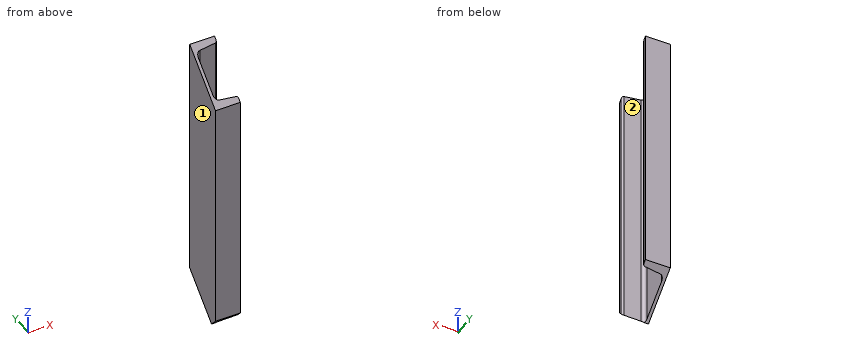
Autodesk Inventor part; units mm, degrees
ref_plane "Начальная плоскость" through (0, 0, 23.4485) normal (0, 0, 1) x (1, 0, 0)
ref_plane "Конечная плоскость" through (0, 0, 422.7409) normal (0, 0, 1) x (1, 0, 0)
ref_plane "РабПлоскость8" through (36, 285.6248, 665.6679) normal (0, -0.6924238, 0.721491) x (1, 0, 0)
ref_plane "Начальная плоскость" through (0, 0, 23.4485) normal (0, 0, 1) x (1, 0, 0)
ref_plane "Конечная плоскость" through (0, 0, 422.7409) normal (0, 0, 1) x (1, 0, 0)
sketch "Эскиз" plane through (0, 0, 0) normal (0, 0, 1) x (1, 0, 0)
  line L0 (36, -32.5) -> (0, -32.5)
  line L1 (36, -32.5) -> (36, -28.696)
  line L2 (33.6994, -26.2039) -> (9.9215, -24.3017)
  line L3 (4.4, -18.3208) -> (4.4, 18.3208)
  line L4 (33.6994, 26.2039) -> (9.9215, 24.3017)
  line L5 (36, 28.696) -> (36, 32.5)
  line L6 (0, 32.5) -> (36, 32.5)
  line L7 (0, -32.5) -> (0, 32.5)
  arc A0 (4.4, -18.3208) -> (9.9215, -24.3017) centre (10.4, -18.3208) ccw
  arc A1 (9.9215, 24.3017) -> (4.4, 18.3208) centre (10.4, 18.3208) ccw
  arc A2 (36, -28.696) -> (33.6994, -26.2039) centre (33.5, -28.696) ccw
  arc A3 (33.6994, 26.2039) -> (36, 28.696) centre (33.5, 28.696) ccw
  line L8 (0, 45.5) -> (0, -45.5) construction
  line L9 (-7.2974, 0) -> (43.7847, 0) construction
  point P0 (36, -26.388)
  point P1 (4.4, -23.86)
  point P2 (4.4, 23.86)
  point P3 (36, 26.388)
  dimension "d3" = 36
  dimension "d5" = 4.4
  dimension "d7" = 65
  dimension "d9" = 8.64
  dimension "d11" = 8.64
  dimension "d13" = 6.112
  dimension "d15" = 6.112
  dimension "d22" = 6
  dimension "d23" = 2.5
  dimension "d24" = 32.5
  dimension "d25" = 0
extrude "Тело" add sketch "Эскиз" along normal up to surface (399.2924 mm away) from surface at 23.4485
sketch "Sketch3" plane through (0, 0, 0) normal (0, 0, 1) x (1, 0, 0)
  line L0 (0, 0) -> (10, 0)
ref_plane "Work Plane7" through (0, 0, 0) normal (0, -1, 0) x (1, 0, 0)
sketch "Sketch4" plane through (0, 0, 0) normal (0, -1, 0) x (1, 0, 0)
  line L0 (-2, 23.4485) -> (12, 23.4485)
  line L1 (-2, 422.7409) -> (12, 422.7409)
  dimension "d29" = 399.2924
ref_plane "РабПлоскость8" through (36, 285.6248, 665.6679) normal (0, -0.6924238, 0.721491) x (1, 0, 0)
split "Разделение1" plane through (36, 285.6248, 665.6679) removes the side toward (0, -0.6924238, 0.721491)
ref_plane "РабПлоскость9" through (0, 458.7307, 485.2951) normal (0, 0.6924238, -0.721491) x (1, 0, 0)
split "Разделение2" plane through (0, 458.7307, 485.2951) removes the side toward (0, 0.6924238, -0.721491)
ref_plane "РабПлоскость10" through (36, 195.6464, -203.8595) normal (0, -0.721491, -0.6924238) x (1, 0, 0)
split "Разделение3" plane through (36, 195.6464, -203.8595) removes the side toward (0, -0.721491, -0.6924238)
equation "\"d3\" = b"
equation "\"d7\" = ParH"
equation "\"d22\" = R"
equation "\"d23\" = R1"
equation "\"d24\" = 0.5 * d7"
equation "\"d16\" = G_L"
equation "\"R1\" = 2.5"
equation "\"R\" = 6"
equation "\"t1\" = 4.4"
equation "\"t2\" = 7.2"
equation "\"ParH\" = 65"
equation "\"b\" = 36"
equation "\"msp_x1\" = 0.04 * b"
equation "\"msp_x2\" = -0.08 * t1 + 0.04 * b"
equation "\"G_L\" = d29"
equation "\"ex\" = 0"
equation "\"G_OFFSET_START\" = -23.44846"
equation "\"G_OFFSET_END\" = -58.90056"
equation "\"d26\" = -G_OFFSET_START"
equation "\"d27\" = G_OFFSET_END + B_L"
equation "\"B_L\" = 481.64146"
properties part number "Швеллер 6.5U-399,29 ГОСТ 8240-97" material "Сталь, мягкая"
CAD build for the part. Positions are in the model's coordinates, mm. Face numbers are marked on the shaded views. A direction names the side the tool comes from. Coordinates: 2 decimals unless noted, no trailing zeros. Write each loop counter-clockwise with the first axis right and the second up, starting at its lowest first coordinate (ties: lowest second). Pieces come first, ordered by that corner, then holes. Notation, with made-up numbers: M 51.5,6.5 L 102.5,6.5 A20 ccw 102.5,43.5 Z; hole C 29.25,-29 d3. An arc over 180 degrees is marked long. Answer as a JSON object with one key per item and string values. Group by question number.
1) Saw through at C-C (z = 392.5). Write the cut outline in (x, y), plus the area to 3 significant figures.
2) Saw through at B-B (z = 150). Write the cut outline in (x, y), plus the area to 3 significant figures.
3) Saw through at D-D (y = 10.5). Write the cut outline in (x, z).
4) Tool access for the marked faces 1 and 2: list every direction of +Z, -Z, +X, -X, +Y, -Y with a clear straight run to the whole face (end or side of a thin tool).
5) Saw through at A-A (x = 18.5). Write the cut outline in (y, z), plus the area to 3 significant figures.
6) Wall check: line 1 (Y direction, x = 33, z = 325); line 2 (X direction, y = 1, z = 314.5); line 3 (Y direction, x = 33, z = 385.5). Give the ranges that are in metal, low to high. Write a range as from..to.
7) Pin check, flat tip, straight feed: pin 1 Ø2 at (x, y) = (5, -24.5) entering from +Z. Stop position of the tip, or through.
Values follow:
{
 "1": {"outline": "M 0,0.99 L 4.4,0.99 L 4.4,18.32 A6 cw 9.92,24.3 L 33.7,26.2 A2.5 ccw 36,28.7 L 36,32.5 L 0,32.5 Z", "area": "377 mm2"},
 "2": {"outline": "M 0,-32.5 L 36,-32.5 L 36,-28.7 A2.5 ccw 33.7,-26.2 L 9.92,-24.3 A6 cw 4.4,-18.32 L 4.4,18.32 A6 cw 9.92,24.3 L 33.7,26.2 A2.5 ccw 36,28.7 L 36,32.5 L 0,32.5 Z", "area": "763 mm2"},
 "3": {"outline": "M 0,55.12 L 4.4,55.12 L 4.4,401.63 L 0,401.63 Z"},
 "4": {"face 1": "+Z, -Z, -X, +Y, -Y", "face 2": "+Z, -Z, +X"},
 "5": {"outline": "M -32.5,33.86 L -24.99,26.04 L -24.99,367.57 L -32.5,360.36 Z; M 24.99,69.03 L 32.5,76.24 L 32.5,422.74 L 24.99,415.53 Z", "area": "5,110 mm2"},
 "6": {"line 1": "y = -32.5..-26.15, 26.15..32.5", "line 2": "x = 0..4.4", "line 3": "y = 26.15..32.5"},
 "7": {"pin 1": "stops at z = 369"}
}
